```python
from build123d import *

# Parameters (mm, degrees)
SKETCH4_W           = 70
SKETCH4_H           = 40
BOSS_EXTRUDE3_DEPTH = 44
SKETCH5_W           = 38
SKETCH5_H           = 40
CUT_EXTRUDE5_DEPTH  = 92.847700026
CUT_EXTRUDE8_DEPTH  = 92.847700026
CHAMFER2_SIZE       = 3
SKETCH9_R           = 5
CUT_EXTRUDE9_DEPTH  = 92.847700026


with BuildPart() as part:
    # Sketch4 → Boss-Extrude3 (new body)
    with BuildSketch(Plane(origin=(0, 0, 0), x_dir=(1, 0, 0), z_dir=(0, 1, 0))):
        with Locations((35, 20)):
            Rectangle(SKETCH4_W, SKETCH4_H)
    extrude(amount=BOSS_EXTRUDE3_DEPTH)

    # Sketch5 → Cut-Extrude5 (cut, through all)
    with BuildSketch(Plane.ZY):
        with Locations((-21, 22)):
            Rectangle(SKETCH5_W, SKETCH5_H)
    extrude(amount=-CUT_EXTRUDE5_DEPTH, mode=Mode.SUBTRACT)

    # Sketch8 → Cut-Extrude8 (cut, through all)
    with BuildSketch(Plane(origin=(0, 44, 0), x_dir=(1, 0, 0), z_dir=(0, 1, 0))):
        Polygon((10, 40), (55, 15), (70, 0), (70, 40), align=None)
    extrude(amount=-CUT_EXTRUDE8_DEPTH, mode=Mode.SUBTRACT)

    # Chamfer2
    chamfer2_edges = [part.edges().sort_by_distance(p)[0] for p in [
        (0, 1, -40),
        (0, 43, -40),
    ]]
    chamfer(chamfer2_edges, length=CHAMFER2_SIZE)

    # Sketch9 → Cut-Extrude9 (cut, through all)
    with BuildSketch(Plane(origin=(0, 44, 0), x_dir=(1, 0, 0), z_dir=(0, 1, 0))):
        with Locations(Location((8, 32, 0), (0, 0, 270))):
            Circle(SKETCH9_R)
        with Locations(Location((16, 8, 0), (0, 0, 270))):
            Circle(SKETCH9_R)
    extrude(amount=-CUT_EXTRUDE9_DEPTH, mode=Mode.SUBTRACT)


solid = part.part
```
Geometry check sheet. Reference: the model listing, model coordinates, mm. A direction names the side the tool comes from. Coordinates: 2 decimals unless noted, no trailing zeros. Loops run counter-clockwise (first coordinate to the right, second up) from the corner with the lowest first, then second, coordinate; pieces in that order, holes last. Notation, with made-up numbers: (65.25, 88) - (112.25, 88) arc R26 ccw to (112.25, 109) - close; hole circle Ø4 at (64, 62). An arc over 180 degrees is marked (long way). One line per item, written item: value. Start each with the question number.
(1) Cross-section at D-D on x = 66. Enter the section's corners in (y, z).
(2) Depth check by flat-ended pin: P1, Ø3, axis at x = 57.5, y = 6, coming from the -Z side. Enter the tip coordinate at first touch or a pass-through.
(3) Cross-section at A-A on z = -18.5. Enter the section's corners in (x, y).
(4) Cross-section at C-C on z = -32. Enter the section's corners in (x, y).
(5) Material ranges on line 1 (Y direction, x = 14, z = -32); line 2 (Z direction, x = 24.5, y = 8); line 3 (X direction, y = 1, z = -32), recorded low to high. Write a range as [from, to].
(6) Mould release check, pull along Y, two halves, no side actions. Record for faces 1 (the flat face through (6, 1, -40)), 2 (the flat face through (27, 0, -16)), 3 (the flat face through (26, 2, -17)): released by +Y, released by -Y, zero draft, split by the parting line, or undercut.
(7) Tool access check on faces 4 (the cylindrical face through (11.564, 1.014, -5.693)), 5 (the flat face through (34, 22, -2)). Record the directions out of +Z, -Z, +X, -X, +Y, -Y that give a thin tool (end or side, any length) a straight path to the whole face; none if there is none.
(8) Cross-section at B-B on x = 8. Enter the section's corners in (y, z).
Results below:
1. outline: (0, -4) - (2, -4) - (2, -2) - (42, -2) - (42, -4) - (44, -4) - (44, 0) - (0, 0) - close
2. P1: stops at z = -2
3. outline: (0, 0) - (48.7, 0) - (48.7, 2) - (0, 2) - close; (0, 42) - (48.7, 42) - (48.7, 44) - (0, 44) - close
4. outline: (0, 0) - (3, 0) - (3, 2) - (0, 2) - close; (0, 42) - (3, 42) - (3, 44) - (0, 44) - close; (13, 0) - (24.4, 0) - (24.4, 2) - (13, 2) - close; (13, 42) - (24.4, 42) - (24.4, 44) - (13, 44) - close
5. line 1: y = [0, 2], [42, 44]
5. line 2: z = [-2, 0]
5. line 3: x = [0, 3], [13, 24.4]
6. face 1: zero draft
6. face 2: released by -Y
6. face 3: undercut
7. face 4: +Y, -Y
7. face 5: -Z, +X, -X
8. outline: (0, -40) - (2, -40) - (2, -37) - (0, -37) - close; (0, -27) - (2, -27) - (2, -2) - (42, -2) - (42, -27) - (44, -27) - (44, 0) - (0, 0) - close; (42, -40) - (44, -40) - (44, -37) - (42, -37) - close
